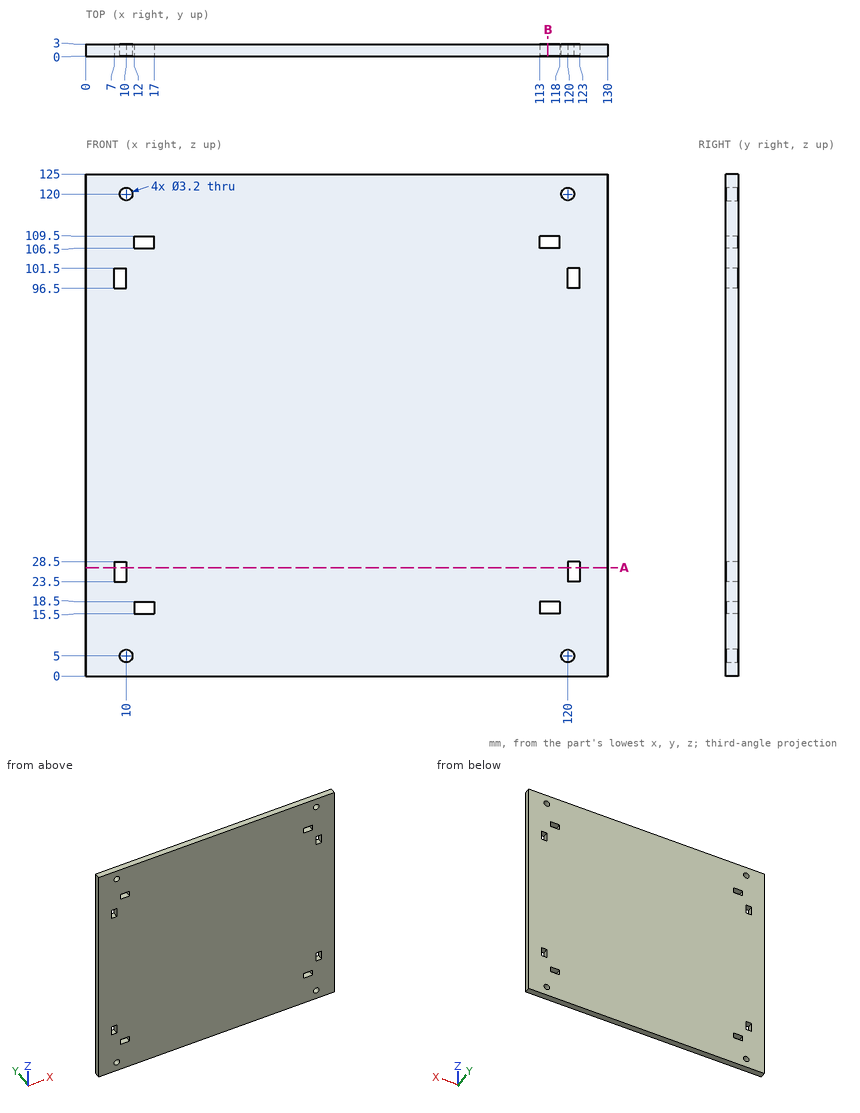
Print and shaded views of the part. All mm, measured from the part's lowest x, y and z. Coordinates: 2 decimals unless noted, no trailing zeros. Write each loop counter-clockwise with the first axis right and the second up, starting at its lowest first coordinate (ties: lowest second). Pieces come first, ordered by that corner, then holes. Notation, with made-up numbers: (56, 8.5) -> (79, 8.5) arc R9 ccw to (79, 20.5) -> close; hole circle Ø4 at (83.5, -25). An arc over 180 degrees is marked (long way). Use CSV: the item, a comma, the result in double quotes. Start each with the question number.
Q1. Cut at B-B, the plane x = 115. List the corners of the cut face in (y, z), then the cut area to 3 significant figures.
Q2. Drill centre lines: probe 1 along Z at (x, y) = (115, 0.55); probe 2 along X at (y, z) = (1.75, 5). Where is each one in solid material? Low to high.
Q3. Cut at A-A, the plane z = 27. List the corners of the cut face in (x, y).
Checked values:
1,outline,"(0, 0) -> (3, 0) -> (3, 15.5) -> (0, 15.5) -> close; (0, 18.5) -> (3, 18.5) -> (3, 106.5) -> (0, 106.5) -> close; (0, 109.5) -> (3, 109.5) -> (3, 125) -> (0, 125) -> close"
1,area,"357 mm²"
2,probe 1,"z = 0 to 15.5, 18.5 to 106.5, 109.5 to 125"
2,probe 2,"x = 0 to 8.4, 11.6 to 118.4, 121.6 to 130"
3,outline,"(0, 0) -> (7, 0) -> (7, 3) -> (0, 3) -> close; (10, 0) -> (120, 0) -> (120, 3) -> (10, 3) -> close; (123, 0) -> (130, 0) -> (130, 3) -> (123, 3) -> close"
